The listing builds one solid part. Answer for the finished solid, in the listing's coordinates (mm). Give positions to 0.01 mm unless a question says otherwise; leave off trailing zeros. Use a Markdown table: item, result. Add a question column.
1) The mould has two halves that part along Z. Classify faces 1 (the face through (-7, -148, -10)), 2 (the face through (-7, -148, 10)), 3 (the face through (0.1, 0, 2.4)), 4 (the face through (-4.5, -148, 0)): released by +Z, released by -Z, zero draft, split by the parting line, or undercut.
2) Straight lines are drawn through the part: line 1 (X direction, y = -88, z = -7.5); line 2 (Z direction, x = 0, y = -106.5); line 3 (X direction, y = -264, z = -5). For each, find the intervals that lie inside material, in ascending order.
3) Flat-ended cylindrical pins translate along their axes: pin 1 (5.5 mm diameter, centred on y = -131, z = 1, fed in from +X); pin 2 (2 mm diameter, centred on x = -0.5, y = -144, fed in from -Z); pin 3 (5.5 mm diameter, centred on y = -100, z = 1, fed in from -X). Find the tip coordinate at first contact, or state that the pin passes through.
from build123d import *

# Parameters (mm, degrees)
SKETCH_R  = 2.1
PAD_DEPTH = 300


with BuildPart() as part:
    # Sketch → Pad (new body)
    with BuildSketch(Plane.XZ):
        with BuildLine():
            Line((-8.2, 5.5), (-8.2, 3.1))
            Line((-10, 4.1), (-8.2, 3.1))
            Line((-10, 4.1), (-10, 9.5))
            ThreePointArc((-9.5, 10), (-9.853553, 9.853553), (-10, 9.5))
            Line((-9.5, 10), (-4.1, 10))
            Line((-4.1, 10), (-3.1, 8.2))
            Line((-3.1, 8.2), (-5.5, 8.2))
            Line((-5.5, 8.2), (-5.5, 6.56066))
            Line((-3.43934, 4.5), (-5.5, 6.56066))
            Line((3.43934, 4.5), (-3.43934, 4.5))
            Line((5.5, 6.56066), (3.43934, 4.5))
            Line((5.5, 8.2), (5.5, 6.56066))
            Line((3.1, 8.2), (5.5, 8.2))
            Line((3.1, 8.2), (4.9, 10))
            Line((4.9, 10), (9.5, 10))
            ThreePointArc((10, 9.5), (9.853553, 9.853553), (9.5, 10))
            Line((10, 9.5), (10, 4.9))
            Line((10, 4.9), (8.2, 3.1))
            Line((8.2, 3.1), (8.2, 5.5))
            Line((8.2, 5.5), (6.56066, 5.5))
            Line((6.56066, 5.5), (4.5, 3.43934))
            Line((4.5, 3.43934), (4.5, -3.43934))
            Line((4.5, -3.43934), (6.56066, -5.5))
            Line((6.56066, -5.5), (8.2, -5.5))
            Line((8.2, -5.5), (8.2, -3.1))
            Line((8.2, -3.1), (10, -4.1))
            Line((10, -4.1), (10, -9.5))
            ThreePointArc((9.5, -10), (9.853553, -9.853553), (10, -9.5))
            Line((4.1, -10), (9.5, -10))
            Line((4.1, -10), (3.1, -8.2))
            Line((3.1, -8.2), (5.5, -8.2))
            Line((5.5, -8.2), (5.5, -6.56066))
            Line((5.5, -6.56066), (3.43934, -4.5))
            Line((-3.43934, -4.5), (3.43934, -4.5))
            Line((-5.5, -6.56066), (-3.43934, -4.5))
            Line((-5.5, -6.56066), (-5.5, -8.2))
            Line((-5.5, -8.2), (-3.2, -8.2))
            Line((-3.2, -8.2), (-4.9, -10))
            Line((-4.9, -10), (-9.5, -10))
            ThreePointArc((-10, -9.5), (-9.853553, -9.853553), (-9.5, -10))
            Line((-10, -9.5), (-10, -4.9))
            Line((-10, -4.9), (-8.2, -3.2))
            Line((-8.2, -3.2), (-8.2, -5.5))
            Line((-8.2, -5.5), (-6.56066, -5.5))
            Line((-6.56066, -5.5), (-4.5, -3.43934))
            Line((-4.5, -3.43934), (-4.5, 3.43934))
            Line((-6.56066, 5.5), (-4.5, 3.43934))
            Line((-8.2, 5.5), (-6.56066, 5.5))
        make_face()
        Circle(SKETCH_R, mode=Mode.SUBTRACT)
    extrude(amount=PAD_DEPTH)


solid = part.part
The answers:
| question | item | result |
|---|---|---|
| 1 | face 1 | released by -Z |
| 1 | face 2 | released by +Z |
| 1 | face 3 | zero draft |
| 1 | face 4 | undercut |
| 2 | line 1 | -10 to -5.5, 5.5 to 10 |
| 2 | line 2 | -4.5 to -2.1, 2.1 to 4.5 |
| 2 | line 3 | -10 to -8.2, -6.06 to -3.94, 3.94 to 6.06, 8.2 to 10 |
| 3 | pin 1 | x = 8.85 |
| 3 | pin 2 | z = -4.5 |
| 3 | pin 3 | x = -9.37 |
